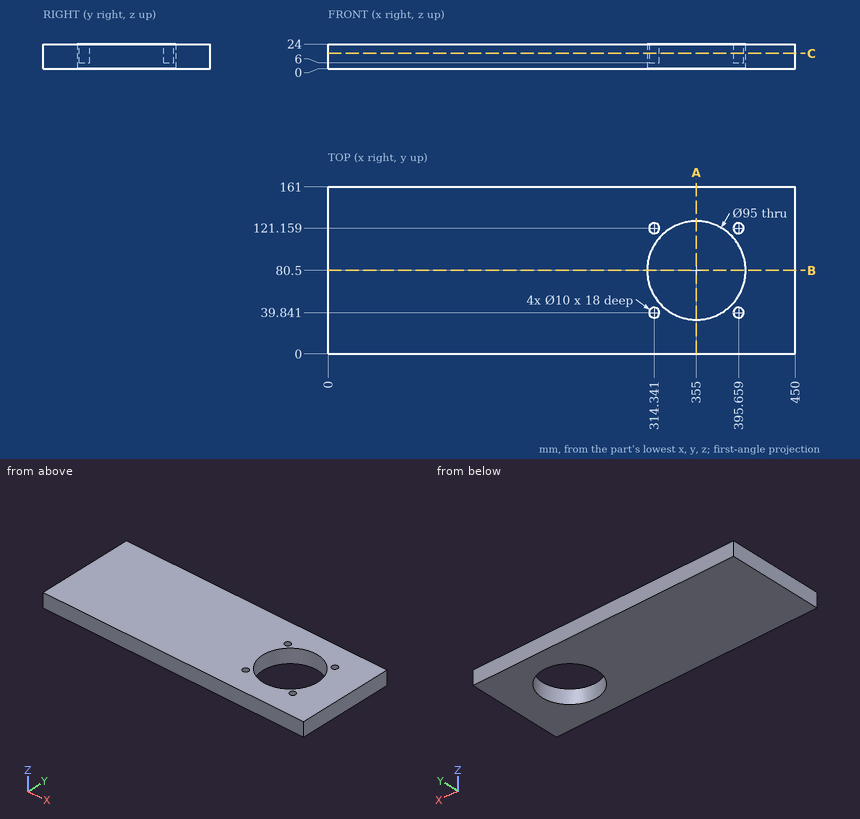
Geometry: see drawing. Coordinates: mm, zero at the bounding-box minimum. Give positions to 0.01 mm unless a question says otherwise; leave off trailing zeros. Order: outer loops, then holes, each group sorted by start corner. A loop starts at its lowest first (then second) coordinate and runs counter-clockwise, first axis right, second up. Notation, with made-up numbers: (6, -13) - (26, -13) arc R13 cw to (26, 1) - close; hole circle Ø3 at (39.5, -2). An arc over 180 degrees is marked (long way). Write each question's results on one line, items separated by ' | '.
Item 1: Section B-B (y = 80.5). Return loops of the section in (x, z).
A:
outline: (0, 0) - (307.5, 0) - (307.5, 24) - (0, 24) - close; (402.5, 0) - (450, 0) - (450, 24) - (402.5, 24) - close
Item 2: Section C-C (z = 15). Return loops of the section in (x, y).
A:
outline: (0, 0) - (450, 0) - (450, 161) - (0, 161) - close; hole circle Ø95 at (355, 80.5); hole circle Ø10 at (314.34, 39.84); hole circle Ø10 at (314.34, 121.16); hole circle Ø10 at (395.66, 39.84); hole circle Ø10 at (395.66, 121.16)
Item 3: Material intervals for line 1 along X through (y, z) = (93.5, 17.75); line 2 along X through (y, z) = (40, 15.75) (1 decimal); line 3 along X through (y, z) = (39, 9.75) (1 decimal), sorted ascending.
A:
line 1: x = 0 to 309.31, 400.69 to 450 | line 2: x = 0 to 309.3, 319.3 to 330.2, 379.8 to 390.7, 400.7 to 450 | line 3: x = 0 to 309.4, 319.3 to 331.9, 378.1 to 390.7, 400.6 to 450
Item 4: Section A-A (x = 355). Return loops of the section in (y, z).
A:
outline: (0, 0) - (33, 0) - (33, 24) - (0, 24) - close; (128, 0) - (161, 0) - (161, 24) - (128, 24) - close
Item 5: Contact query for flat-ended pins moving along their axis: pin 1 Ø16 at (x, y) = (314.34, 121.16) entering from -Z; pin 2 Ø5 at (x, y) = (314, 120) entering from +Z. Output: stop coordinate, or through.
A:
pin 1: stops at z = 0 | pin 2: stops at z = 6
